from build123d import *

# Parameters (mm, degrees)
SKETCH1_W                = 43.18
SKETCH1_H                = 17.78
BOSS_EXTRUDE1_DEPTH      = 1.651
SKETCH2_R                = 0.635
CUT_EXTRUDE1_DEPTH       = 47.726508547
BOSS_EXTRUDE2_DEPTH      = 1.651
BOSS_EXTRUDE2_DEPTH_BACK = 6.35
SKETCH4_W                = 2.54
SKETCH4_H                = 5.08
BOSS_EXTRUDE3_DEPTH      = 1.27
SKETCH5_R                = 0.635
CUT_EXTRUDE2_DEPTH       = 49.378332557
SKETCH6_W                = 2.180271617
SKETCH6_H                = 0.803257964
SKETCH6_H_2              = 0.726757206
SKETCH6_H_3              = 0.688506826
SKETCH6_H_4              = 0.612006068
BOSS_EXTRUDE4_DEPTH      = 0.381


with BuildPart() as part:
    # Sketch1 → Boss-Extrude1 (new body)
    with BuildSketch(Plane(origin=(0, 0, 0), x_dir=(1, 0, 0), z_dir=(0, 1, 0))):
        with Locations((21.59, 8.89)):
            Rectangle(SKETCH1_W, SKETCH1_H)
    extrude(amount=BOSS_EXTRUDE1_DEPTH)

    # Sketch2 → Cut-Extrude1 (cut, through all)
    with BuildSketch(Plane(origin=(0, 1.651, 0), x_dir=(1, 0, 0), z_dir=(0, 1, 0))):
        with Locations(Location((2.54, 1.905, 0), (0, 0, 270))):
            Circle(SKETCH2_R)
        with Locations(Location((5.08, 1.905, 0), (0, 0, 270))):
            Circle(SKETCH2_R)
        with Locations(Location((7.62, 1.905, 0), (0, 0, 270))):
            Circle(SKETCH2_R)
        with Locations(Location((10.16, 1.905, 0), (0, 0, 270))):
            Circle(SKETCH2_R)
        with Locations(Location((12.7, 1.905, 0), (0, 0, 270))):
            Circle(SKETCH2_R)
        with Locations(Location((15.24, 1.905, 0), (0, 0, 270))):
            Circle(SKETCH2_R)
        with Locations(Location((17.78, 1.905, 0), (0, 0, 270))):
            Circle(SKETCH2_R)
        with Locations(Location((20.32, 1.905, 0), (0, 0, 270))):
            Circle(SKETCH2_R)
        with Locations(Location((22.86, 1.905, 0), (0, 0, 270))):
            Circle(SKETCH2_R)
        with Locations(Location((25.4, 1.905, 0), (0, 0, 270))):
            Circle(SKETCH2_R)
        with Locations(Location((27.94, 1.905, 0), (0, 0, 270))):
            Circle(SKETCH2_R)
        with Locations(Location((30.48, 1.905, 0), (0, 0, 270))):
            Circle(SKETCH2_R)
        with Locations(Location((33.02, 1.905, 0), (0, 0, 270))):
            Circle(SKETCH2_R)
        with Locations(Location((35.56, 1.905, 0), (0, 0, 270))):
            Circle(SKETCH2_R)
        with Locations(Location((38.1, 1.905, 0), (0, 0, 270))):
            Circle(SKETCH2_R)
        with Locations(Location((38.1, 15.875, 0), (0, 0, 90))):
            Circle(SKETCH2_R)
        with Locations(Location((35.56, 15.875, 0), (0, 0, 90))):
            Circle(SKETCH2_R)
        with Locations(Location((33.02, 15.875, 0), (0, 0, 90))):
            Circle(SKETCH2_R)
        with Locations(Location((30.48, 15.875, 0), (0, 0, 90))):
            Circle(SKETCH2_R)
        with Locations(Location((27.94, 15.875, 0), (0, 0, 90))):
            Circle(SKETCH2_R)
        with Locations(Location((25.4, 15.875, 0), (0, 0, 90))):
            Circle(SKETCH2_R)
        with Locations(Location((22.86, 15.875, 0), (0, 0, 90))):
            Circle(SKETCH2_R)
        with Locations(Location((20.32, 15.875, 0), (0, 0, 90))):
            Circle(SKETCH2_R)
        with Locations(Location((17.78, 15.875, 0), (0, 0, 90))):
            Circle(SKETCH2_R)
        with Locations(Location((15.24, 15.875, 0), (0, 0, 90))):
            Circle(SKETCH2_R)
        with Locations(Location((12.7, 15.875, 0), (0, 0, 90))):
            Circle(SKETCH2_R)
        with Locations(Location((10.16, 15.875, 0), (0, 0, 90))):
            Circle(SKETCH2_R)
        with Locations(Location((7.62, 15.875, 0), (0, 0, 90))):
            Circle(SKETCH2_R)
        with Locations(Location((5.08, 15.875, 0), (0, 0, 90))):
            Circle(SKETCH2_R)
        with Locations(Location((2.54, 15.875, 0), (0, 0, 90))):
            Circle(SKETCH2_R)
    extrude(amount=-CUT_EXTRUDE1_DEPTH, mode=Mode.SUBTRACT)

    # Sketch3 → Boss-Extrude2 (add, two sides: drawn at the far end of the back side and taken through both)
    with BuildSketch(Plane(origin=(43.18, 0, 0), x_dir=(0, 0, -1), z_dir=(1, 0, 0)).offset(-BOSS_EXTRUDE2_DEPTH_BACK)):
        with BuildLine():
            Line((6.35, 1.651), (11.43, 1.651))
            Line((11.43, 1.651), (11.43, 3.556))
            ThreePointArc((11.43, 3.556), (11.615987194, 4.005012806), (12.065, 4.191))
            Line((12.065, 4.191), (12.446, 4.191))
            ThreePointArc((12.446, 4.191), (12.625605122, 4.265394878), (12.7, 4.445))
            Line((12.7, 4.445), (12.7, 4.953))
            ThreePointArc((12.7, 4.953), (12.551210245, 5.312210245), (12.192, 5.461))
            Line((12.192, 5.461), (5.588, 5.461))
            ThreePointArc((5.588, 5.461), (5.228789755, 5.312210245), (5.08, 4.953))
            Line((5.08, 4.953), (5.08, 4.445))
            ThreePointArc((5.08, 4.445), (5.154394878, 4.265394878), (5.334, 4.191))
            Line((5.334, 4.191), (5.715, 4.191))
            ThreePointArc((5.715, 4.191), (6.164012806, 4.005012806), (6.35, 3.556))
            Line((6.35, 3.556), (6.35, 1.651))
        make_face()
    extrude(amount=BOSS_EXTRUDE2_DEPTH + BOSS_EXTRUDE2_DEPTH_BACK)

    # Sketch4 → Boss-Extrude3 (add)
    with BuildSketch(Plane(origin=(0, 1.651, 0), x_dir=(1, 0, 0), z_dir=(0, 1, 0))):
        Polygon((27.198541148, 8.89), (30.744270574, 12.435729426), (34.29, 8.89), (30.744270574, 5.344270574), align=None)
        with Locations((22.118541148, 8.89)):
            Rectangle(SKETCH4_W, SKETCH4_H)
    extrude(amount=BOSS_EXTRUDE3_DEPTH)

    # Sketch5 → Cut-Extrude2 (cut, through all)
    with BuildSketch(Plane(origin=(0, 1.651, 0), x_dir=(1, 0, 0), z_dir=(0, 1, 0))):
        with Locations(Location((2.54, 11.43, 0), (0, 0, 270))):
            Circle(SKETCH5_R)
        with Locations(Location((5.08, 11.43, 0), (0, 0, 270))):
            Circle(SKETCH5_R)
        with Locations(Location((5.08, 8.89, 0), (0, 0, 270))):
            Circle(SKETCH5_R)
        with Locations(Location((2.54, 8.89, 0), (0, 0, 270))):
            Circle(SKETCH5_R)
        with Locations(Location((2.54, 6.35, 0), (0, 0, 270))):
            Circle(SKETCH5_R)
        with Locations(Location((5.08, 6.35, 0), (0, 0, 270))):
            Circle(SKETCH5_R)
    extrude(amount=-CUT_EXTRUDE2_DEPTH, mode=Mode.SUBTRACT)

    # Sketch6 → Boss-Extrude4 (add)
    with BuildSketch(Plane(origin=(0, 1.651, 0), x_dir=(1, 0, 0), z_dir=(0, 1, 0))):
        with Locations((9.83041316, 11.344327099)):
            Rectangle(SKETCH6_W, SKETCH6_H)
        with Locations((9.83041316, 9.508308895)):
            Rectangle(SKETCH6_W, SKETCH6_H_2)
        with Locations((9.83041316, 7.538414363)):
            Rectangle(SKETCH6_W, SKETCH6_H_3)
        with Locations((9.83041316, 5.281641987)):
            Rectangle(SKETCH6_W, SKETCH6_H_4)
    extrude(amount=BOSS_EXTRUDE4_DEPTH)


solid = part.part
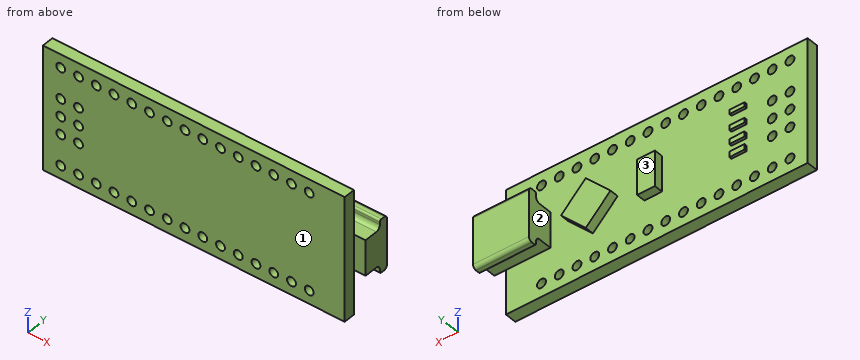
The model under review builds one solid part; all positions refer to its coordinate system, in mm. Face numbers are marked on the shaded views. A direction names the side the tool comes from. Round coordinates to 2 decimals unless told otherwise and drop trailing zeros. Write each loop counter-clockwise with the first axis right and the second up, starting at its lowest first coordinate (ties: lowest second). Pieces come first, ordered by that corner, then holes. Notation, with made-up numbers: (81.25, 14.5) - (138.25, 14.5) arc R14 cw to (138.25, 22.5) - close; hole circle Ø1 at (30.5, 44.5). An arc over 180 degrees is marked (long way). One line per item, written item: value. Start each with the question number.
1. Machinability: for the marked faces 1, 2 and 3, which of the approach directions +Z, -Z, +X, -X, +Y, -Y give a long, thin tool a straight path to every point of the face, cutting with its end or side? Answer none if there is none.
2. Consider section D-D on x = 39.5. Write out the cut boundary in (y, z) (3 decimals).
3. Clearance check with flat-ended pins moving along their axes: P1, Ø0.8, axis at x = 2.54, z = -15.875, coming from the -Y side; P2, Ø1.5, axis at x = 25.4, z = -1.905, coming from the +Y side; P3, Ø5.5, axis at x = 32, z = -6.5, coming from the +Y side; P4, Ø6, axis at x = 7.5, z = -10.5, coming from the +Y side. State where each tip first meets the part, or that it passes through.
4. Consider section C-C on y = 0.6. State how many separate pieces and enclosed holes the cut face has, and give its area (3 significant figures).
5. To check wall thickness, follow L1, parallel to Z at x = 38.1, y = 1.35; L2, parallel to X at y = 0.85, z = -8.89 (3 decimals); L3, parallel to Y at x = 42, z = -12.25. State the ranges of each line that lie inside material, in increasing order. Write a range as from..to.
6. Consider section B-B on x = 25.4. Write out the cut boundary in (y, z).
7. Consider section A-A on x = 2.54. Write out the cut boundary in (y, z) (3 decimals), and give its area (3 significant figures).
Checks:
1. face 1: +Z, -Z, +X, -X, -Y
1. face 2: +Z, -Z, +Y
1. face 3: +Z, -Z, -X, +Y
2. outline: (0, -17.78) - (1.651, -17.78) - (1.651, -11.43) - (3.556, -11.43) arc R0.635 cw to (4.191, -12.065) - (4.191, -12.446) arc R0.254 ccw to (4.445, -12.7) - (4.953, -12.7) arc R0.508 ccw to (5.461, -12.192) - (5.461, -5.588) arc R0.508 ccw to (4.953, -5.08) - (4.445, -5.08) arc R0.254 ccw to (4.191, -5.334) - (4.191, -5.715) arc R0.635 cw to (3.556, -6.35) - (1.651, -6.35) - (1.651, 0) - (0, 0) - close
3. P1: passes through
3. P2: stops at y = 1.65
3. P3: stops at y = 2.92
3. P4: stops at y = 2.03
4. separate pieces: 1
4. enclosed holes: 36
4. area: 722 mm^2
5. L1: z = -17.78..-16.51, -15.24..-2.54, -1.27..0
5. L2: x = 0..1.905, 3.175..4.445, 5.715..43.18
5. L3: y = 0..1.65, 4.19..5.46
6. outline: (0, -17.78) - (1.65, -17.78) - (1.65, -16.51) - (0, -16.51) - close; (0, -15.24) - (1.65, -15.24) - (1.65, -2.54) - (0, -2.54) - close; (0, -1.27) - (1.65, -1.27) - (1.65, 0) - (0, 0) - close
7. outline: (0, -17.78) - (1.651, -17.78) - (1.651, -16.51) - (0, -16.51) - close; (0, -15.24) - (1.651, -15.24) - (1.651, -12.065) - (0, -12.065) - close; (0, -10.795) - (1.651, -10.795) - (1.651, -9.525) - (0, -9.525) - close; (0, -8.255) - (1.651, -8.255) - (1.651, -6.985) - (0, -6.985) - close; (0, -5.715) - (1.651, -5.715) - (1.651, -2.54) - (0, -2.54) - close; (0, -1.27) - (1.651, -1.27) - (1.651, 0) - (0, 0) - close
7. area: 18.9 mm^2
